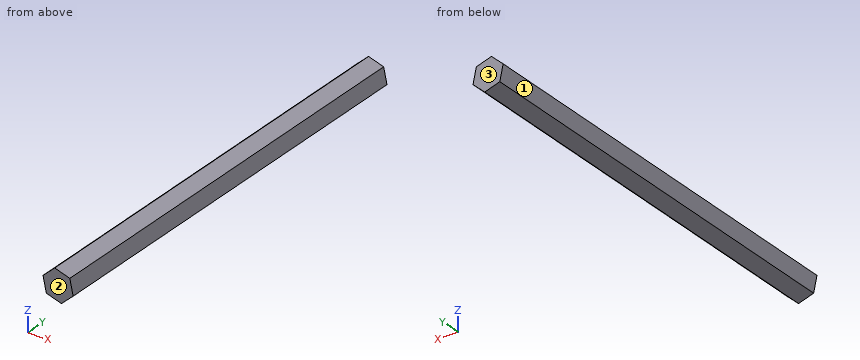
from build123d import *

# Parameters (mm, degrees)
BOSS_EXTRUDE1_DEPTH = 127
SKETCH3_W           = 20.194547067
SKETCH3_H           = 18.170773651
CUT_EXTRUDE1_DEPTH  = 38.1
BOSS_EXTRUDE2_DEPTH = 2.54
SKETCH5_W           = 34.517572909
SKETCH5_H           = 22.340458643
CUT_EXTRUDE2_DEPTH  = 50
BOSS_EXTRUDE3_DEPTH = 25
BOSS_EXTRUDE4_DEPTH = 13.5


with BuildPart() as part:
    # Sketch2 → Boss-Extrude1 (new body)
    with BuildSketch(Plane(origin=(0, 0, 0), x_dir=(1, 0, 0), z_dir=(0, 1, 0))):
        Polygon((2.137295047, -1.940438924), (2.749116926, 0.880732344), (0.611821879, 2.821171268), (-2.137295047, 1.940438924), (-2.749116926, -0.880732344), (-0.611821879, -2.821171268), align=None)
    extrude(amount=BOSS_EXTRUDE1_DEPTH)

    # Sketch3 → Cut-Extrude1 (cut)
    with BuildSketch(Plane.XZ):
        with Locations((-3.121926418, 0.771419978)):
            Rectangle(SKETCH3_W, SKETCH3_H)
    extrude(amount=-CUT_EXTRUDE1_DEPTH, mode=Mode.SUBTRACT)

    # Sketch4 → Boss-Extrude2 (add)
    with BuildSketch(Plane.XZ.offset(-38.1)):
        Polygon((0.611821879, -2.821171268), (2.749116926, -0.880732344), (2.137295047, 1.940438924), (-0.611821879, 2.821171268), (-2.749116926, 0.880732344), (-2.137295047, -1.940438924), align=None)
    extrude(amount=BOSS_EXTRUDE2_DEPTH)

    # Sketch5 → Cut-Extrude2 (cut)
    with BuildSketch(Plane.XZ.offset(-35.56)):
        with Locations((-1.3482575, -1.032578251)):
            Rectangle(SKETCH5_W, SKETCH5_H)
    extrude(amount=-CUT_EXTRUDE2_DEPTH, mode=Mode.SUBTRACT)

    # Sketch7 → Boss-Extrude3 (add)
    with BuildSketch(Plane.XZ.offset(-85.56)):
        Polygon((0.611821879, -2.821171268), (2.749116926, -0.880732344), (2.137295047, 1.940438924), (-0.611821879, 2.821171268), (-2.749116926, 0.880732344), (-2.137295047, -1.940438924), align=None)
    extrude(amount=BOSS_EXTRUDE3_DEPTH)

    # Sketch8 → Boss-Extrude4 (add)
    with BuildSketch(Plane.XZ.offset(-60.56)):
        Polygon((0.611821879, -2.821171268), (2.749116926, -0.880732344), (2.137295047, 1.940438924), (-0.611821879, 2.821171268), (-2.749116926, 0.880732344), (-2.137295047, -1.940438924), align=None)
    extrude(amount=BOSS_EXTRUDE4_DEPTH)


solid = part.part
Can you work these out from the model? Positions are in its coordinate system, mm. Face numbers are marked on the shaded views. Give positions to 0.01 mm unless a question says otherwise; leave off trailing zeros. Loops run counter-clockwise (first coordinate to the right, second up) from the corner with the lowest first, then second, coordinate; pieces in that order, holes last. Notation, with made-up numbers: (36.25, 55) - (72.25, 55) arc R21 cw to (72.25, 79) - close; hole circle Ø10 at (61.25, 71). An arc over 180 degrees is marked (long way). Answer as a JSON object with one key per item and string values.
Q1. Imagine slicing it at A-A on y = 68. Write out the boundary of the cut face in (x, z).
Geometry says:
{"outline": "(-2.75, 0.88) - (-2.14, -1.94) - (0.61, -2.82) - (2.75, -0.88) - (2.14, 1.94) - (-0.61, 2.82) - close"}
Q2. If we mould it in two halves opening along Y, with no side actions, what happens to the marked faces 1, 2 and 3? For each: pulls with the +Y half, pulls with the -Y half, needs draft (parallel to the pull), parting line crosses it, or undercut.
Geometry says:
{"face 1": "needs draft", "face 2": "pulls with the -Y half", "face 3": "pulls with the +Y half"}
Q3. If I drill on L1, parallel to X at y = 97.5, z = 0.05; L2, parallel to X at y = 72, z = 1.45; L3, parallel to Z at x = 2.05, y = 113.5, over which ranges is the centre line in solid material (lowest first)?
Geometry says:
{"L1": "-2.57 to 2.55", "L2": "-2.12 to 2.24", "L3": "-1.52 to 1.97"}
